Could you check a few things on this model? Use its own coordinates, in mm. Face numbers are marked on the shaded views. A direction names the side the tool comes from. Give positions to 0.01 mm unless a question says otherwise; leave off trailing zeros. Loops run counter-clockwise (first coordinate to the right, second up) from the corner with the lowest first, then second, coordinate; pieces in that order, holes last. Notation, with made-up numbers: (10.5, -6) -> (58.5, -6) arc R16 ccw to (58.5, 1) -> close; hole circle Ø7 at (48, -7). An arc over 180 degrees is marked (long way). Write item = value, one per line. Start each with the question number.
1) I want a section at D-D (x = -6.75). List the corners of the cut face in (y, z) for me.
2) On a 3-axis mill with a long thin cutter (end or side, diameter ignored), from which of +Z, -Z, +X, -X, +Y, -Y can I reach the whole of each face in a straight line? I mean the marked faces 1, 2 and 3. Say none if no direction works.
3) I'm going to push flat-ended pins straight in: pin 1 Ø8.5 at (x, y) = (2.5, 4) entering from +Z; pin 2 Ø1.9 at (x, y) = (0.5, -4) entering from +Z (3 decimals); pin 3 Ø1 at (x, z) = (2.5, 10) entering from +Y; pin 4 Ø2 at (y, z) = (5, 11) entering from +X. Where does each tip first touch, or does it pass through?
4) I need wall thicknesses on probe 1 along Z at (x, y) = (-1.5, -5) (3 decimals); probe 2 along Z at (x, y) = (1, 2); probe 3 along Z at (x, y) = (4.25, -3) (3 decimals). Which ranges of each line are inside material? Lowest first, please. Write a range as from..to.
5) I want a section at A-A (x = 0). Count the separate pieces of the cut face and the enclosed holes in it, and give its area (3 significant figures).
from build123d import *

# Parameters (mm, degrees)
F0_R     = 8.255
F1_DEPTH = 2.54
F8_DEPTH = 33.656
F9_W     = 6.078346395
F9_H     = 6.078346395
F10_W    = 5.8075642901
F10_H    = 5.8075642901


# Not quite as in the source:
# - a pattern or mirror of a feature is missing from the dataset's text; its kind, count and spacing are read off the source's solid


with BuildPart() as f1:
    # F0 (on Top) → F1 (new body)
    with BuildSketch(Plane.XY):
        Circle(F0_R)
    extrude(amount=F1_DEPTH)

    # F2 (on Top) → F5 section 0
    with BuildSketch(Plane.XY):
        Polygon((4.7625, 2.3625), (4.7625, 4.7625), (2.3625, 4.7625), (-2.3625, 4.7625), (-4.7625, 4.7625), (-4.7625, 2.3625), (-4.7625, -2.3625), (-4.7625, -4.7625), (-2.3625, -4.7625), (2.3625, -4.7625), (4.7625, -4.7625), (4.7625, -2.3625), align=None)
    # F4 (on offset) → F5 section 1
    with BuildSketch(Plane.XY.offset(19.05)):
        Polygon((-3.4371664787, 5.8371664787), (-5.8371664787, 5.8371664787), (-5.8371664787, 3.4371664787), (-5.8371664787, -3.4371664787), (-5.8371664787, -5.8371664787), (-3.4371664787, -5.8371664787), (3.4371664787, -5.8371664787), (5.8371664787, -5.8371664787), (5.8371664787, -3.4371664787), (5.8371664787, 3.4371664787), (5.8371664787, 5.8371664787), (3.4371664787, 5.8371664787), align=None)
    loft()

    # F7 (on offset) → F8 (cut, through all)
    with BuildSketch(Plane.XZ.offset(25.4)):
        Polygon((3.0391731975, 11.995), (3.4371664787, 19.05), (-3.4371664787, 19.05), (-3.0391731975, 11.995), align=None)
        Polygon((-2.5057888638, 2.54), (2.5057888638, 2.54), (2.903782145, 9.595), (-2.903782145, 9.595), align=None)
    f8 = extrude(amount=-F8_DEPTH, mode=Mode.SUBTRACT)

    # F8_copies: F8 across plane
    add(f8.mirror(Plane(origin=(0, 0, 0), x_dir=(0.7071067812, -0.7071067812, 0), z_dir=(0.7071067812, 0.7071067812, 0))), mode=Mode.SUBTRACT)

    # F9 (on face) → F11 section 0
    with BuildSketch(Plane.XY.offset(11.995)):
        Rectangle(F9_W, F9_H)
    # F10 (on face) → F11 section 1
    with BuildSketch(Plane(origin=(0, 0, 9.595), x_dir=(1, 0, 0), z_dir=(0, 0, -1))):
        Rectangle(F10_W, F10_H)
    loft(mode=Mode.SUBTRACT)


solid = f1.part
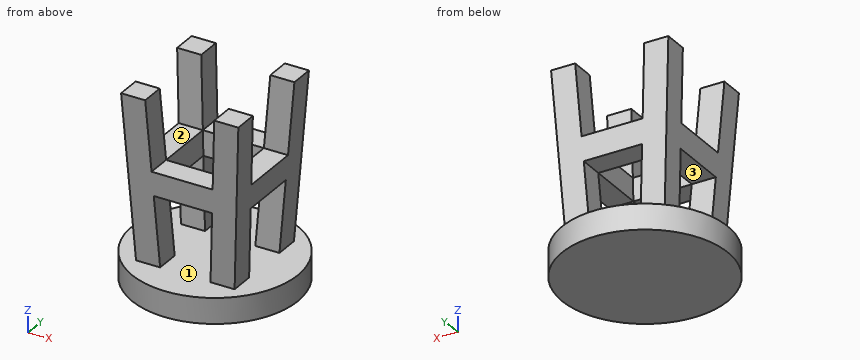
Answer list:
q1.outline = (-4.75, 0) -> (4.75, 0) -> (4.75, 2.54) -> (-4.75, 2.54) -> close
q2.face_1 = none
q2.face_2 = +Z, +X, -X
q2.face_3 = +X, -X
q3.pin_1 = 19.05
q3.pin_2 = 11.995
q3.pin_3 = 5.35
q3.pin_4 = 5.44
q4.probe_1 = 0..2.54, 9.595..11.995
q4.probe_2 = 0..2.54
q4.probe_3 = 0..11.995
q5.separate_pieces = 3
q5.enclosed_holes = 0
q5.area = 53.5 mm^2
